The model under review builds one solid part; all positions refer to its coordinate system, in mm. Face numbers are marked on the shaded views. A direction names the side the tool comes from. Coordinates: 2 decimals unless noted, no trailing zeros. Loops run counter-clockwise (first coordinate to the right, second up) from the corner with the lowest first, then second, coordinate; pieces in that order, holes last. Notation, with made-up numbers: M 19.25,-8.75 L 59.25,-8.75 A6 ccw 59.25,-4.75 Z; hole C 80.25,-36.5 d8. An arc over 180 degrees is marked long. Write item = value, one per line. Start each with the question number.
Q1. For the marked faces 1 and 2, list the 3-axis set-ups (+Z, -Z, +X, -X, +Y, -Y) from which the entire face can be reached by the end or side of a thin tool; tool diameter is ignored.
Q2. Wall thickness on probe 1 along X at (y, z) = (21, -12); probe 2 along Z at (x, y) = (-11.75, 24.5); probe 3 along X at (y, z) = (15.5, 4.75): over which ranges is each line inside the solid? List them lowest first.
Q3. We need section A-A on x = 0. Give the boundary of the cut face in (y, z).
Q4. Mouldability with a two-part tool opening along X and no side actions: class the marked faces 3, 4, 5 and 6 as released by +X, released by -X, zero draft, split by the parting line, or undercut.
Q5. We need section B-B on z = 7.5. Give the boundary of the cut face in (x, y), and give its area (3 significant figures).
Q6. Clearance check with flat-ended pins moving along their axes: pin 1 Ø12 at (x, z) = (-11, 3) entering from -Y; pin 2 Ø7 at (x, y) = (0, 2) entering from +Z; pin 3 Ø2.5 at (y, z) = (-4, -1) entering from +X. State where each tip first meets the part, or that it passes through.
Q7. We need section C-C on y = 9.5. Count the separate pieces of the cut face and the enclosed holes in it, and give its area (3 significant figures).
Autodesk Fusion 360 part; units mm, degrees
sketch "Sketch1" plane through (0, 0, 0) normal (0, 1, 0) x (1, 0, 0)
  circle A0 centre (0, 0) radius 3.4
  line L0 (15, -15) -> (4.5, -15)
  line L1 (4.5, -15) -> (4.5, -14.5)
  line L2 (4.5, -14.5) -> (4, -14.5)
  line L3 (4, -14.5) -> (4, -13)
  line L4 (4, -13) -> (9, -13)
  line L5 (15, -15) -> (15, -4.5)
  line L6 (15, -4.5) -> (14.5, -4.5)
  line L7 (14.5, -4.5) -> (14.5, -4)
  line L8 (14.5, -4) -> (13, -4)
  line L9 (13, -4) -> (13, -9)
  line L10 (13, -9) -> (10.4142, -9)
  line L11 (9, -13) -> (9, -10.4142)
  line L12 (9, -10.4142) -> (4.5858, -6)
  line L13 (10.4142, -9) -> (6, -4.5858)
  line L14 (13, 4) -> (13, 9)
  line L15 (14.5, 4) -> (13, 4)
  line L16 (9, 10.4142) -> (4.5858, 6)
  line L17 (15, 4.5) -> (14.5, 4.5)
  line L18 (4.5, 15) -> (4.5, 14.5)
  line L19 (4, 14.5) -> (4, 13)
  line L20 (10.4142, 9) -> (6, 4.5858)
  line L21 (13, 9) -> (10.4142, 9)
  line L22 (15, 15) -> (4.5, 15)
  line L23 (4, 13) -> (9, 13)
  line L24 (4.5, 14.5) -> (4, 14.5)
  line L25 (15, 15) -> (15, 4.5)
  line L26 (14.5, 4.5) -> (14.5, 4)
  line L27 (9, 13) -> (9, 10.4142)
  line L28 (-4, 13) -> (-9, 13)
  line L29 (-4, 14.5) -> (-4, 13)
  line L30 (-10.4142, 9) -> (-6, 4.5858)
  line L31 (-4.5, 15) -> (-4.5, 14.5)
  line L32 (-15, 4.5) -> (-14.5, 4.5)
  line L33 (-14.5, 4) -> (-13, 4)
  line L34 (-9, 10.4142) -> (-4.5858, 6)
  line L35 (-9, 13) -> (-9, 10.4142)
  line L36 (-15, 15) -> (-15, 4.5)
  line L37 (-13, 4) -> (-13, 9)
  line L38 (-14.5, 4.5) -> (-14.5, 4)
  line L39 (-15, 15) -> (-4.5, 15)
  line L40 (-4.5, 14.5) -> (-4, 14.5)
  line L41 (-13, 9) -> (-10.4142, 9)
  line L42 (-13, -4) -> (-13, -9)
  line L43 (-14.5, -4) -> (-13, -4)
  line L44 (-9, -10.4142) -> (-4.5858, -6)
  line L45 (-15, -4.5) -> (-14.5, -4.5)
  line L46 (-4.5, -15) -> (-4.5, -14.5)
  line L47 (-4, -14.5) -> (-4, -13)
  line L48 (-10.4142, -9) -> (-6, -4.5858)
  line L49 (-13, -9) -> (-10.4142, -9)
  line L50 (-15, -15) -> (-4.5, -15)
  line L51 (-4, -13) -> (-9, -13)
  line L52 (-4.5, -14.5) -> (-4, -14.5)
  line L53 (-15, -15) -> (-15, -4.5)
  line L54 (-14.5, -4.5) -> (-14.5, -4)
  line L55 (-9, -13) -> (-9, -10.4142)
  line L56 (4.5858, -6) -> (-4.5858, -6)
  line L57 (-6, -4.5858) -> (-6, 4.5858)
  line L58 (-4.5858, 6) -> (4.5858, 6)
  line L59 (6, 4.5858) -> (6, -4.5858)
  circle A1 centre (12, -12) radius 1.5
  circle A2 centre (12, 12) radius 1.5
  circle A3 centre (-12, 12) radius 1.5
  circle A4 centre (-12, -12) radius 1.5
  dimension "d1" = 6.8
  dimension "d7" = 360
  dimension "d8" = 3
  dimension "d9" = 8
  dimension "d10" = 30
  dimension "d11" = 12
  dimension "d22" = 18
  dimension "d23" = 2
  dimension "d24" = 7
extrude "Extrude1" add sketch "Sketch1" along normal mid plane 100
fillet "Fillet1" radius 0.5 4 edges at (-15, 0, 15) (15, 0, 15) (-15, 0, -15) (15, 0, -15)
fillet "Fillet2" radius 0.3 8 edges at (-13, 0, -9) (-9, 0, -13) (9, 0, -13) (13, 0, -9) (13, 0, 9) (9, 0, 13) (-9, 0, 13) (-13, 0, 9)
fillet "Fillet3" radius 0.3 8 edges at (-10.4142, 0, -9) (-9, 0, -10.4142) (9, 0, -10.4142) (10.4142, 0, -9) (-9, 0, 10.4142) (-10.4142, 0, 9) (9, 0, 10.4142) (10.4142, 0, 9)
fillet "Fillet4" radius 0.5 8 edges at (-4.5858, 0, 6) (6, 0, 4.5858) (6, 0, -4.5858) (4.5858, 0, 6) (-6, 0, 4.5858) (-6, 0, -4.5858) (4.5858, 0, -6) (-4.5858, 0, -6)
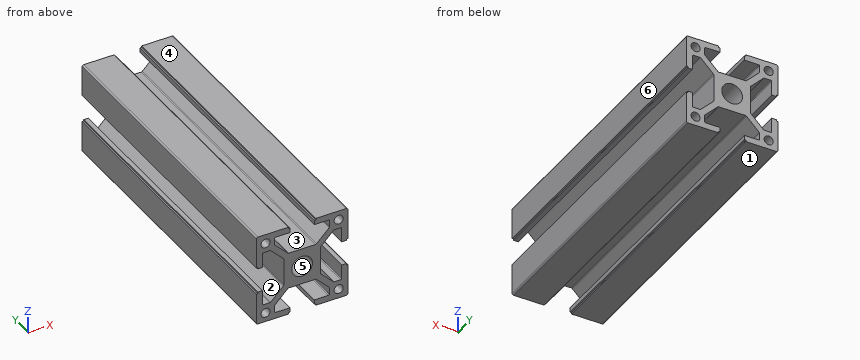
Returned:
q1.face_1 = -Z, +X, -X, +Y, -Y
q1.face_2 = +Y, -Y
q2.probe_1 = -15 to -13.5, -10.5 to -9, 9 to 10.5, 13.5 to 15
q2.probe_2 = -15 to -13.48, -10.52 to -9, 9 to 10.52, 13.48 to 15
q2.probe_3 = -15 to -13, -6.16 to 6.16, 13 to 15
q3.outline = M -50,-6 L 50,-6 L 50,-3.4 L -50,-3.4 Z; M -50,3.4 L 50,3.4 L 50,6 L -50,6 Z
q4.face_3 = undercut
q4.face_4 = zero draft
q4.face_5 = undercut
q4.face_6 = released by +X
q5.outline = M -15,-50 L -13,-50 L -13,50 L -15,50 Z; M -8.91,-50 L -6.09,-50 L -6.09,50 L -8.91,50 Z; M 6.09,-50 L 8.91,-50 L 8.91,50 L 6.09,50 Z; M 13,-50 L 15,-50 L 15,50 L 13,50 Z
q5.area = 966 mm^2
q6.pin_1 = -50
q6.pin_2 = 6
q6.pin_3 = 6
q7.separate_pieces = 1
q7.enclosed_holes = 5
q7.area = 343 mm^2
